Part model, mm, in its own coordinate system. Face numbers are marked on the shaded views. Coordinates: 2 decimals unless noted, no trailing zeros. Loops run counter-clockwise (first coordinate to the right, second up) from the corner with the lowest first, then second, coordinate; pieces in that order, holes last. Notation, with made-up numbers: (-9.75, -36) -> (11.25, -36) arc R15 cw to (11.25, -17) -> close; hole circle Ø2 at (38, 24.25). An arc over 180 degrees is marked (long way). One line per item, written item: value. Start each with the question number.
from build123d import *

# Parameters (mm, degrees)
BASE_FLANGE1_DEPTH = 16.66875
SKETCH2_R          = 2.54
CUT_EXTRUDE1_DEPTH = 2.54
SKETCH3_R          = 2.54
CUT_EXTRUDE2_DEPTH = 1.5875


# Sheet-metal steps are written as plain solids
with BuildPart() as part:
    # Sketch1 → Base-Flange1 (new, symmetric)
    with BuildSketch(Plane.XY):
        with BuildLine():
            Line((0, 0), (46.423806115, 17.477308657))
            ThreePointArc((46.423806115, 17.477308657), (47.542459326, 17.680904949), (48.661112536, 17.477308657))
            Line((48.661112536, 17.477308657), (95.084918652, 0))
            Line((95.084918652, 0), (94.525592046, -1.485701854))
            Line((94.525592046, -1.485701854), (48.101785931, 15.991606803))
            ThreePointArc((48.101785931, 15.991606803), (47.542459326, 16.093404949), (46.983132721, 15.991606803))
            Line((46.983132721, 15.991606803), (0.559326605, -1.485701854))
            Line((0.559326605, -1.485701854), (0, 0))
        make_face()
    extrude(amount=BASE_FLANGE1_DEPTH, both=True)

    # Sketch2 → Cut-Extrude1 (cut)
    with BuildSketch(Plane(origin=(0, 0, 0), x_dir=(0.9358751835780662, 0.3523317197794163, 0), z_dir=(-0.3523317197794163, 0.9358751835780662, 0))):
        with Locations(Location((13.536698287, 0, 0), (0, 0, 180))):
            Circle(SKETCH2_R)
    extrude(amount=-CUT_EXTRUDE1_DEPTH, mode=Mode.SUBTRACT)

    # Sketch3 → Cut-Extrude2 (cut)
    with BuildSketch(Plane(origin=(11.803617474, 31.353159678, 0), x_dir=(0.9358751835780662, -0.3523317197794163, 0), z_dir=(0.3523317197794163, 0.9358751835780662, 0))):
        with Locations(Location((76.541615699, 0, 0), (0, 0, 180))):
            Circle(SKETCH3_R)
    extrude(amount=-CUT_EXTRUDE2_DEPTH, mode=Mode.SUBTRACT)


solid = part.part
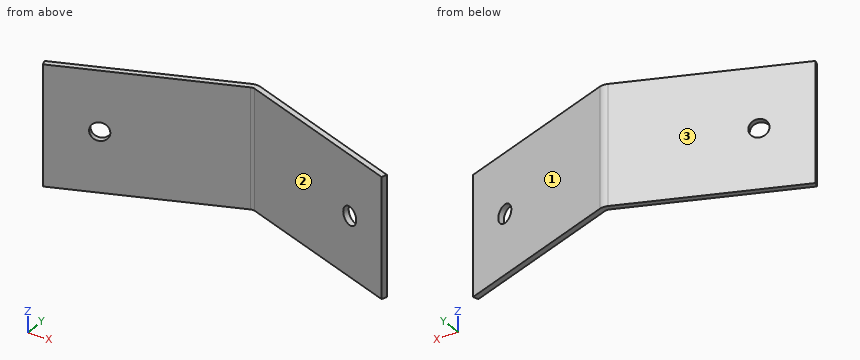
1) Pin check, flat tips, straight feed: pin 1 Ø1 at (x, z) = (12, -4.5) entering from -Y; pin 2 Ø4 at (x, z) = (54, -5) entering from -Y; pin 3 Ø1.5 at (x, z) = (37.5, 13) entering from +Y. Stop position of each tip, or through.
2) Slice it at C-C (x = 24). Give the cut face in (y, z).
3) Probe line 1 (Y direction, x = 59, z = 11) (3 decimals); line 2 (Y direction, x = 9, z = 15.5). List the from-to ranges inside material, lowest first. Write a range as from..to.
4) Slice it at A-A (y = 8.5). Give the cut face in (x, z).
5) Pull direction X, two halves, no side cores. Call the marked faces 1, 2 and 3: +X half, -X half, draft (parallel to the pull), parting line (faces both ways), or undercut.
Check sheet entries:
1. pin 1: stops at y = 2.63
1. pin 2: stops at y = 13.02
1. pin 3: stops at y = 14.4
2. outline: (7.34, -16.67) -> (9.04, -16.67) -> (9.04, 16.67) -> (7.34, 16.67) -> close
3. line 1: y = 11.889..13.585
3. line 2: y = 1.69..3.39
4. outline: (22.58, -16.67) -> (27.08, -16.67) -> (27.08, 16.67) -> (22.58, 16.67) -> close; (68, -16.67) -> (72.51, -16.67) -> (72.51, 16.67) -> (68, 16.67) -> close
5. face 1: +X half
5. face 2: undercut
5. face 3: -X half
